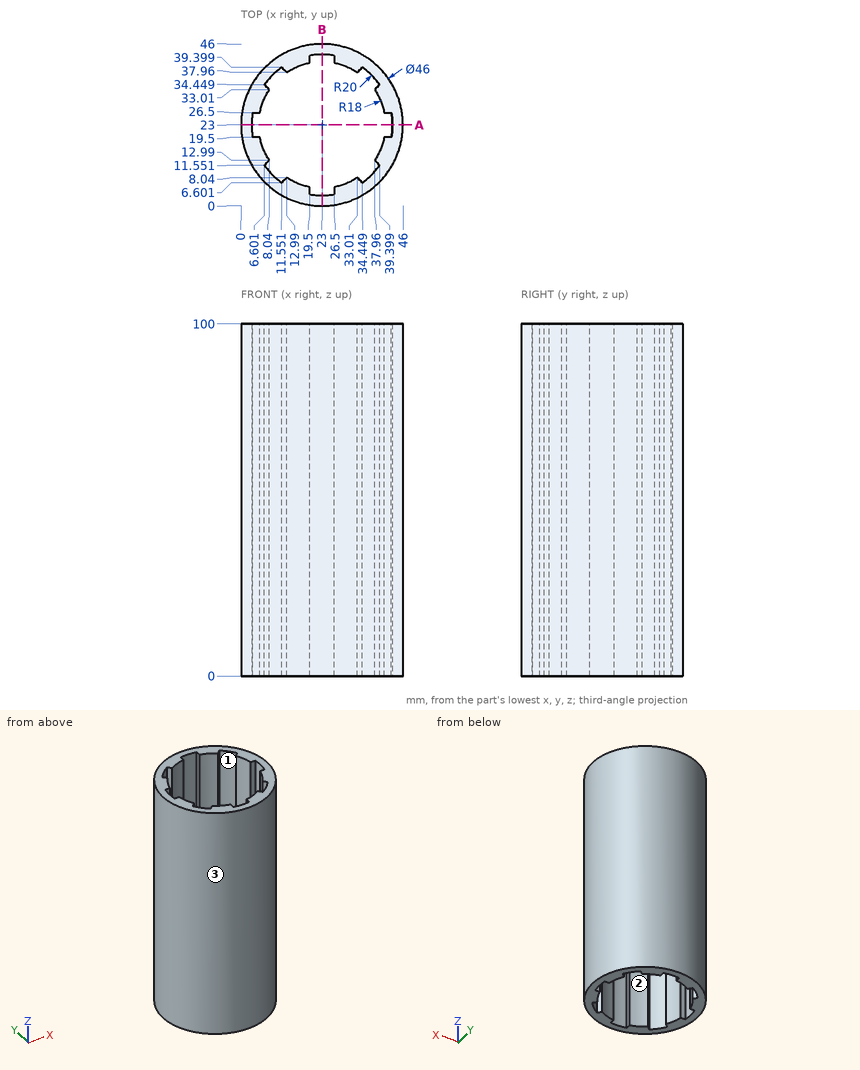
The drawing under review shows one solid part. Ordinate dimensions are in mm from its lowest x, y, z. Round coordinates to 2 decimals unless told otherwise and drop trailing zeros. Loops run counter-clockwise (first coordinate to the right, second up) from the corner with the lowest first, then second, coordinate; pieces in that order, holes last. Notation, with made-up numbers: (87, 44.25) -> (133, 44.25) arc R25 cw to (133, 78.25) -> close; hole circle Ø7 at (-27.5, -26.5). An arc over 180 degrees is marked (long way). One line per question, with ' | ' between items. Start each with the question number.
Item 1: For pin 1 (1.5 mm diameter, centred on y = 34.5, z = 22.5, fed in from -X); pin 2 (2 mm diameter, centred on y = 4.5, z = 69.5, fed in from +X) (1 decimal); pin 3 (1.5 mm diameter, centred on y = 30.5, z = 33, fed in from +X), all flat-tipped, find the tip position at first contact; note any pin that passes through.
Item 2: Wall thickness on line 1 along X through (y, z) = (31.5, 92); line 2 along X through (y, z) = (36, 19.5); line 3 along Y through (x, z) = (19, 91): over which ranges is each line inside the solid? List them lowest first. Write a range as [from, to].
Item 3: Add section A-A, the plane y = 23. Write out the cut boundary in (x, z), then the cut area to 3 significant figures.
Item 4: Draft analysis for pull direction X (two halves, no side actions). For the marked faces 1, 2 and 3, state which applies: +X half, -X half, draft (parallel to the pull), parting line (faces both ways), or undercut.
Return value:
1) pin 1: stops at x = 2.67 | pin 2: stops at x = 37.9 | pin 3: stops at x = 44.99
2) line 1: x = [1.63, 7.13], [38.87, 44.37] | line 2: x = [4.03, 7.8], [38.2, 41.97] | line 3: y = [0.35, 5.45], [40.55, 45.65]
3) outline: (0, 0) -> (3, 0) -> (3, 100) -> (0, 100) -> close; (43, 0) -> (46, 0) -> (46, 100) -> (43, 100) -> close | area: 600 mm2
4) face 1: undercut | face 2: undercut | face 3: parting line
